```python
from build123d import *

# Parameters (mm, degrees)
PAD_DEPTH       = 30
SKETCH001_R     = 1.8
SKETCH001_W     = 29.168577
SKETCH001_H     = 18
POCKET_DEPTH    = 15.001
SKETCH002_R     = 2.8
POCKET001_DEPTH = 30.001


with BuildPart() as part:
    # Sketch → Pad (new body)
    with BuildSketch(Plane.XY):
        Polygon((-10, 4), (-26, 4), (-26, 0), (0, 0), (0, 15), (-10, 15), align=None)
    extrude(amount=PAD_DEPTH)

    # Sketch001 → Pocket (cut, through all)
    with BuildSketch(Plane.XZ):
        with Locations((-16, 27)):
            Circle(SKETCH001_R)
        with Locations((-16, 3)):
            Circle(SKETCH001_R)
        with Locations((-8.415712, 15)):
            Rectangle(SKETCH001_W, SKETCH001_H)
    extrude(amount=-POCKET_DEPTH, mode=Mode.SUBTRACT)

    # Sketch002 → Pocket001 (cut, through all)
    with BuildSketch(Plane.XY.offset(30)):
        with Locations((-5, 11)):
            Circle(SKETCH002_R)
    extrude(amount=-POCKET001_DEPTH, mode=Mode.SUBTRACT)


solid = part.part
```
Work out the finished part from the listing and answer in its coordinate system (mm). A direction names the side the tool comes from. Give positions to 0.01 mm unless a question says otherwise; leave off trailing zeros. Loops run counter-clockwise (first coordinate to the right, second up) from the corner with the lowest first, then second, coordinate; pieces in that order, holes last. Notation, with made-up numbers: (46, 89) -> (101, 89) arc R24 ccw to (101, 118) -> close; hole circle Ø8 at (57.5, -5). An arc over 180 degrees is marked (long way). Write item = value, one per line. Start each with the question number.
(1) Find section B-B on z = 27. Give the vertices of the cut face in (x, y), and give its area (3 significant figures).
(2) The mould has two halves that part along X. Classify faces 1 (the flat face through (-7, 6, 0)), 2 (the flat face through (0, 7, 27)), 3 (the cylindrical face through (-3.49, 13.36, 27.04)): +X half, -X half, draft (parallel to the pull), parting line (faces both ways), or undercut.
(3) Find section D-D on y = 6. Give the vertices of the cut face in (x, z), and give its area (3 significant figures).
(4) Find the intervals of material crossed by probe 1 along Z at (x, y) = (-2.5, 13); probe 2 along Z at (x, y) = (-14.5, 3.5); probe 3 along X at (y, z) = (5.75, 3), in increasing order. Write a range as from..to.
(5) Which of the six approach directions +Z, -Z, +X, -X, +Y, -Y give full straight-line access (tool end or side, diameter ignored) to faces 4 (the cylindrical face through (-16.234, 1.972, 4.785)), 5 (the flat face through (-9, 6, 6)), 6 (the flat face through (-23.2, 4, 14.8))?
(6) Find section A-A on x = -16. Give the vertices of the cut face in (y, z), and give its area (3 significant figures).
(7) Given pin 1 Ø1.8 at (y, z) = (10, 27.5) entering from -X; pin 2 Ø7.5 at (x, y) = (-5, 11) entering from +Z; pin 3 Ø4.5 at (x, z) = (-16, 3) entering from +Y; pin 4 Ø3 at (y, z) = (1.5, 18.5) entering from +X, each flat-ended and moving along its own axis, determine where each tip first touches the part or whether it passes through.
(8) Find section C-C on x = -20.75. Give the vertices of the cut face in (y, z), and give its area (3 significant figures).
From the geometry:
q1.outline = (-26, 0) -> (-17.8, 0) -> (-17.8, 4) -> (-26, 4) -> close; (-14.2, 0) -> (0, 0) -> (0, 15) -> (-10, 15) -> (-10, 4) -> (-14.2, 4) -> close; hole circle Ø5.6 at (-5, 11)
q1.area = 175 mm^2
q2.face_1 = draft
q2.face_2 = +X half
q2.face_3 = undercut
q3.outline = (-10, 0) -> (0, 0) -> (0, 6) -> (-10, 6) -> close; (-10, 24) -> (0, 24) -> (0, 30) -> (-10, 30) -> close
q3.area = 120 mm^2
q4.probe_1 = 0..6, 24..30
q4.probe_2 = 0..2.01, 3.99..6, 24..26.01, 27.99..30
q4.probe_3 = -10..0
q5.face_4 = +Y, -Y
q5.face_5 = +X, +Y, -Y
q5.face_6 = +Z, -Z, -X, +Y
q6.outline = (0, 0) -> (4, 0) -> (4, 1.2) -> (0, 1.2) -> close; (0, 4.8) -> (4, 4.8) -> (4, 6) -> (0, 6) -> close; (0, 24) -> (4, 24) -> (4, 25.2) -> (0, 25.2) -> close; (0, 28.8) -> (4, 28.8) -> (4, 30) -> (0, 30) -> close
q6.area = 19.2 mm^2
q7.pin_1 = -10
q7.pin_2 = 30
q7.pin_3 = 4
q7.pin_4 = -23
q8.outline = (0, 0) -> (4, 0) -> (4, 6) -> (0, 6) -> close; (0, 24) -> (4, 24) -> (4, 30) -> (0, 30) -> close
q8.area = 48.0 mm^2
